Read the model definition and answer for the solid it produces. Units are mm, in the model's axes. A direction names the side the tool comes from. Round coordinates to 2 decimals unless told otherwise and drop trailing zeros. Write each loop counter-clockwise with the first axis right and the second up, starting at its lowest first coordinate (ties: lowest second). Pieces come first, ordered by that corner, then holes.
from build123d import *

# Parameters (mm, degrees)
PAD_DEPTH    = 2
PAD001_DEPTH = 2


with BuildPart() as part:
    # Sketch → Pad (new body)
    with BuildSketch(Plane.XY):
        with BuildLine():
            ThreePointArc((24, 15), (0, 39), (-24, 15))
            Line((-24, 15), (-24, -15))
            ThreePointArc((-24, -15), (0, -39), (24, -15))
            Line((24, -15), (24, 15))
        make_face()
        with BuildLine():
            ThreePointArc((21, 15), (0, 36), (-21, 15))
            Line((-21, 15), (-21, -15))
            ThreePointArc((-21, -15), (0, -36), (21, -15))
            Line((21, -15), (21, 15))
        make_face(mode=Mode.SUBTRACT)
    extrude(amount=PAD_DEPTH)

    # Sketch001 (on Face9 of Pad) → Pad001 (join)
    with BuildSketch(Plane(origin=(0, 0, 0), x_dir=(1, 0, 0), z_dir=(0, 0, -1))):
        with BuildLine():
            ThreePointArc((27, 15), (0, 42), (-27, 15))
            Line((-27, 15), (-27, -15))
            ThreePointArc((-27, -15), (0, -42), (27, -15))
            Line((27, -15), (27, 15))
        make_face()
        with BuildLine():
            ThreePointArc((21, 15), (0, 36), (-21, 15))
            Line((-21, 15), (-21, -15))
            ThreePointArc((-21, -15), (0, -36), (21, -15))
            Line((21, -15), (21, 15))
        make_face(mode=Mode.SUBTRACT)
    extrude(amount=PAD001_DEPTH)


solid = part.part
Q1. Section B-B (y = 7) is taken. Determine the outline of the cut face in (x, z), then the cut area to 3 significant figures.
Verdict:
outline: (-27, -2) - (-21, -2) - (-21, 2) - (-24, 2) - (-24, 0) - (-27, 0) - close; (21, -2) - (27, -2) - (27, 0) - (24, 0) - (24, 2) - (21, 2) - close
area: 36.0 mm2
Q2. Flat-ended cylindrical pins translate along their axes: pin 1 Ø1 at (x, z) = (-14, 0) entering from +Y; pin 2 Ø1 at (x, z) = (2, -0.5) entering from -Y; pin 3 Ø2 at (y, z) = (26.5, -1) entering from +X. Find the tip coordinate at first contact, or state that the pin passes through.
Verdict:
pin 1: stops at y = 38.38
pin 2: stops at y = -41.96
pin 3: stops at x = 24.87
Q3. Section C-C (z = -1.35) is taken. Determine the outline of the cut face in (x, y).
Verdict:
outline: (-27, -15) arc R27 ccw to (27, -15) - (27, 15) arc R27 ccw to (-27, 15) - close; hole (-21, -15) arc R21 ccw to (21, -15) - (21, 15) arc R21 ccw to (-21, 15) - close
Q4. Which of the six approach directions +Z, -Z, +X, -X, +Y, -Y give full straight-line access (tool end or side, diameter ignored) to faces 1 (the flat face through (21, 0, 0)), 2 (the cylindrical face through (-0.528, -38.994, 0.986)), 3 (the flat face through (-24, 0, 1)), 4 (the flat face through (24, 0, 1))?
Verdict:
face 1: +Z, -Z
face 2: +Z, -Y
face 3: +Z, -X, +Y, -Y
face 4: +Z, +X, +Y, -Y
Q5. Straight lines are drawn through the part: probe 1 along X at (y, z) = (-15, -0.65); probe 2 along X at (y, z) = (5, 0.45); probe 3 along Y at (x, z) = (0, 0.1). For each, find the intervals that lie inside material, in ascending order.
Verdict:
probe 1: x = -27 to -21, 21 to 27
probe 2: x = -24 to -21, 21 to 24
probe 3: y = -39 to -36, 36 to 39
Q6. Determine the mould class of faces 5 (the cylindrical face through (0, -36, 0)), 6 (the cylindrical face through (0.528, 38.994, 0.986)), 7 (the flat face through (-22, 0, -2)) for opening direction Y: pulls with the +Y half, pulls with the -Y half, needs draft (parallel to the pull), parting line crosses it, or undercut.
Verdict:
face 5: undercut
face 6: pulls with the +Y half
face 7: needs draft
Q7. Section A-A (x = 0) is taken. Determine the outline of the cut face in (y, z), then the cut area to 3 significant figures.
Verdict:
outline: (-42, -2) - (-36, -2) - (-36, 2) - (-39, 2) - (-39, 0) - (-42, 0) - close; (36, -2) - (42, -2) - (42, 0) - (39, 0) - (39, 2) - (36, 2) - close
area: 36.0 mm2
